Check sheet for the modelled part. Datum: model origin and axes. Units: mm. A direction names the side the tool comes from. Give positions to 0.01 mm unless a question says otherwise; leave off trailing zeros. Loops run counter-clockwise (first coordinate to the right, second up) from the corner with the lowest first, then second, coordinate; pieces in that order, holes last. Notation, with made-up numbers: (9, 5.25) -> (54, 5.25) arc R24 cw to (54, 38.25) -> close; hole circle Ø5 at (15.25, 4). An arc over 180 degrees is marked (long way). Write each question's results on one line, items separated by ' | '. Start each with the question number.
Item 1: Mould release check, pull along X, two halves, no side actions. Record for faces 1 (the face through (73.11, 0.164, -48.295)), 2 (the face through (0.724, 0.515, -49.236)), 3 (the face through (40, 0, -25)): pulls with the +X half, pulls with the -X half, needs draft (parallel to the pull), parting line crosses it, or undercut.
Item 2: Cross-section at A-A on x = 16.4. Enter the section's corners in (y, z).
Item 3: Cross-section at B-B on y = 0.5. State how many separate pieces and enclosed holes the cut face has, then the cut area to 3 significant figures.
Item 4: Gauge pin test, flat ends, axial feed: pin 1 Ø2.5 at (x, z) = (73, -4.5) entering from -Y; pin 2 Ø22 at (x, z) = (14.5, -38.5) entering from -Y. Record the tip position at first contact, or that the pin passes through.
Item 5: Access from +Z, -Z, +X, -X, +Y, -Y to the whole of each face (thin tool, end or side, straight path). Record for faces 4 (the face through (4, 0.333, -4)), 5 (the face through (77.236, 0.515, -0.724)).
Item 6: Scan lines: line 1 along Z through (x, y) = (16.4, 0.45); line 2 along Z through (x, y) = (49.5, 0.25); line 3 along Z through (x, y) = (7.5, 0.3). Record each from-to range of solid material in increasing order.
Item 7: Cross-section at C-C on z = -19. Enter the section's corners in (x, y), then the cut area to 3 significant figures.
from build123d import *

# Parameters (mm, degrees)
SKETCH1_W                   = 78
SKETCH1_H                   = 50
STEEL_FACE_DEPTH            = 1.016
CARD_EDGES_R                = 2.54
SKETCH2_R                   = 2.54
MAGNET_CAVITY_DEPTH         = 0.333375
MIRROR2_COPY_1_SKETCH_R     = 2.54
MIRROR2_COPY_1_DEPTH        = 0.333375
SKETCH3_R                   = 10.049999966
BATTERY_POCKETS_DEPTH       = 0.873000032
SKETCH5_W                   = 35.000000104
SKETCH5_H                   = 3.000000096
LED_SLOT_DEPTH              = 93.655449144
LED_SLOT_CORNER_ROUND_R     = 1.27
LED_SLOT_SURFACE_ROUND_R    = 0.127
SKETCH6_W                   = 2.59999988
SKETCH6_H                   = 3.000000096
ALS_DATA_SENSOR_SLOT_DEPTH  = 93.655449144
SKETCH8_W                   = 2.59999988
SKETCH8_H                   = 3.000000096
ALS_CLOCK_SENSOR_SLOT_DEPTH = 93.655449144
FILLET4_SIZE                = 1.27


with BuildPart() as part:
    # Sketch1 → steel_face (new body)
    with BuildSketch(Plane(origin=(0, 0, 0), x_dir=(1, 0, 0), z_dir=(0, 1, 0))):
        with Locations((39, 25)):
            Rectangle(SKETCH1_W, SKETCH1_H)
    extrude(amount=STEEL_FACE_DEPTH)

    # card_edges
    card_edges_edges = [part.edges().sort_by_distance(p)[0] for p in [
        (0, 0.508, -50),
        (78, 0.508, -50),
        (78, 0.508, 0),
        (0, 0.508, 0),
    ]]
    fillet(card_edges_edges, radius=CARD_EDGES_R)

    # Sketch2 → magnet_cavity (cut)
    with BuildSketch(Plane.XZ):
        with Locations(Location((4.1275, -45.8725, 0), (0, 0, 270))):
            Circle(SKETCH2_R)
    magnet_cavity = extrude(amount=-MAGNET_CAVITY_DEPTH, mode=Mode.SUBTRACT)

    # Mirror1: magnet_cavity across plane
    add(magnet_cavity.mirror(Plane.XY.offset(-25.000000038)), mode=Mode.SUBTRACT)

    # Mirror2: magnet_cavity across plane
    add(magnet_cavity.mirror(Plane(origin=(38.999999978, 0, 0), x_dir=(0, 0, 1), z_dir=(1, 0, 0))), mode=Mode.SUBTRACT)

    # Mirror2 copy 1 sketch → Mirror2 copy 1 (cut)
    with BuildSketch(Plane(origin=(77.999999956, 0, -50.000000076), x_dir=(-1, 0, 0), z_dir=(0, -1, 0))):
        with Locations(Location((4.1275, -45.8725, 0), (0, 0, 270))):
            Circle(MIRROR2_COPY_1_SKETCH_R)
    extrude(amount=-MIRROR2_COPY_1_DEPTH, mode=Mode.SUBTRACT)

    # Sketch3 → battery_pockets (cut)
    with BuildSketch(Plane.XZ):
        with Locations(Location((16.399999966, -11.637499966, 0), (0, 0, 270))):
            Circle(SKETCH3_R)
        with Locations(Location((16.399999966, -38.362500034, 0), (0, 0, 270))):
            Circle(SKETCH3_R)
    extrude(amount=-BATTERY_POCKETS_DEPTH, mode=Mode.SUBTRACT)

    # Sketch5 → led_slot (cut, through all)
    with BuildSketch(Plane(origin=(0, 0, 0), x_dir=(1, 0, 0), z_dir=(0, 1, 0))):
        with Locations((58.912499948, 25.000000038)):
            Rectangle(SKETCH5_W, SKETCH5_H)
    extrude(amount=LED_SLOT_DEPTH, mode=Mode.SUBTRACT)

    # led_slot_corner_round
    led_slot_corner_round_edges = [part.edges().sort_by_distance(p)[0] for p in [
        (76.4125, 0.508, -23.49999999),
        (76.4125, 0.508, -26.500000086),
        (41.412499896, 0.508, -26.500000086),
        (41.412499896, 0.508, -23.49999999),
    ]]
    fillet(led_slot_corner_round_edges, radius=LED_SLOT_CORNER_ROUND_R)

    # led_slot_surface_round
    led_slot_surface_round_edges = [part.edges().sort_by_distance(p)[0] for p in [
        (58.912499948, 1.016, -26.500000086),
        (41.412499896, 1.016, -25.000000038),
        (58.912499948, 1.016, -23.49999999),
        (76.4125, 1.016, -25.000000038),
        (41.784474284, 1.016, -26.128025698),
        (41.784474284, 1.016, -23.871974378),
        (76.040525612, 1.016, -26.128025698),
        (76.040525612, 1.016, -23.871974378),
    ]]
    fillet(led_slot_surface_round_edges, radius=LED_SLOT_SURFACE_ROUND_R)

    # Sketch6 → als_data_sensor_slot (cut, through all)
    with BuildSketch(Plane.XZ):
        with Locations((2.88749994, -25.000000038)):
            Rectangle(SKETCH6_W, SKETCH6_H)
    extrude(amount=-ALS_DATA_SENSOR_SLOT_DEPTH, mode=Mode.SUBTRACT)

    # Sketch8 → als_clock_sensor_slot (cut, through all)
    with BuildSketch(Plane.XZ):
        with Locations((36.112500038, -25.000000038)):
            Rectangle(SKETCH8_W, SKETCH8_H)
    extrude(amount=-ALS_CLOCK_SENSOR_SLOT_DEPTH, mode=Mode.SUBTRACT)

    # Fillet4
    # a fillet whose section is not a circle: 1.27 mm, written as the material it adds along each edge
    with BuildSketch(Plane(origin=(1.5875, 0, -26.500000086), x_dir=(0, 0, 1), z_dir=(0, 1, 0)), Plane(origin=(1.5875, 0, -23.49999999), x_dir=(1, 0, 0), z_dir=(0, 1, 0)), Plane(origin=(34.812500098, 0, -23.49999999), x_dir=(1, 0, 0), z_dir=(0, 1, 0))) as fillet4_piece_1:
        with BuildLine():
            add(Edge.make_bspline([(FILLET4_SIZE, 0), (FILLET4_SIZE * 0.831801948466, 0), (FILLET4_SIZE * 0.663603896932, 0), (FILLET4_SIZE * 0.292893218813, FILLET4_SIZE * 0.0716919198361), (FILLET4_SIZE * 0.0716919198361, FILLET4_SIZE * 0.292893218813), (0, FILLET4_SIZE * 0.663603896932), (0, FILLET4_SIZE * 0.831801948466), (0, FILLET4_SIZE)], knots=[0, 0, 0, 0, 0, 0, 0.5, 0.5, 1, 1, 1, 1, 1, 1], degree=5))
            Line((0, FILLET4_SIZE), (-FILLET4_SIZE * 0.02, FILLET4_SIZE))
            Line((-FILLET4_SIZE * 0.02, FILLET4_SIZE), (-FILLET4_SIZE * 0.02, -FILLET4_SIZE * 0.02))
            Line((-FILLET4_SIZE * 0.02, -FILLET4_SIZE * 0.02), (FILLET4_SIZE, -FILLET4_SIZE * 0.02))
            Line((FILLET4_SIZE, -FILLET4_SIZE * 0.02), (FILLET4_SIZE, 0))
        make_face()
    extrude(amount=1.016)
    with BuildSketch(Plane(origin=(4.18749988, 0, -26.500000086), x_dir=(0, 0, 1), z_dir=(0, 1, 0)), Plane(origin=(4.18749988, 0, -23.49999999), x_dir=(-1, 0, 0), z_dir=(0, 1, 0)), Plane(origin=(34.812500098, 0, -26.500000086), x_dir=(1, 0, 0), z_dir=(0, 1, 0)), Plane(origin=(37.412499978, 0, -26.500000086), x_dir=(0, 0, 1), z_dir=(0, 1, 0)), Plane(origin=(37.412499978, 0, -23.49999999), x_dir=(-1, 0, 0), z_dir=(0, 1, 0))) as fillet4_piece_2:
        with BuildLine():
            add(Edge.make_bspline([(FILLET4_SIZE, 0), (FILLET4_SIZE * 0.831801948466, 0), (FILLET4_SIZE * 0.663603896932, 0), (FILLET4_SIZE * 0.292893218813, -FILLET4_SIZE * 0.0716919198361), (FILLET4_SIZE * 0.0716919198361, -FILLET4_SIZE * 0.292893218813), (0, -FILLET4_SIZE * 0.663603896932), (0, -FILLET4_SIZE * 0.831801948466), (0, -FILLET4_SIZE)], knots=[0, 0, 0, 0, 0, 0, 0.5, 0.5, 1, 1, 1, 1, 1, 1], degree=5))
            Line((0, -FILLET4_SIZE), (-FILLET4_SIZE * 0.02, -FILLET4_SIZE))
            Line((-FILLET4_SIZE * 0.02, -FILLET4_SIZE), (-FILLET4_SIZE * 0.02, FILLET4_SIZE * 0.02))
            Line((-FILLET4_SIZE * 0.02, FILLET4_SIZE * 0.02), (FILLET4_SIZE, FILLET4_SIZE * 0.02))
            Line((FILLET4_SIZE, FILLET4_SIZE * 0.02), (FILLET4_SIZE, 0))
        make_face()
    extrude(amount=1.016)


solid = part.part
Answer sheet:
1) face 1: undercut | face 2: pulls with the -X half | face 3: needs draft
2) outline: (0, -50) -> (1.02, -50) -> (1.02, 0) -> (0, 0) -> (0, -1.59) -> (0.87, -1.59) -> (0.87, -21.69) -> (0, -21.69) -> (0, -28.31) -> (0.87, -28.31) -> (0.87, -48.41) -> (0, -48.41) -> close
3) separate pieces: 1 | enclosed holes: 5 | area: 3,140 mm²
4) pin 1: stops at y = 0.33 | pin 2: stops at y = 0
5) face 4: -Y | face 5: +Z, +X, +Y, -Y
6) line 1: z = -50 to -48.41, -28.31 to -21.69, -1.59 to 0 | line 2: z = -50 to -26.5, -23.5 to 0 | line 3: z = -50 to -43.03, -33.69 to -16.31, -6.97 to 0
7) outline: (0, 0) -> (9.56, 0) -> (9.56, 0.87) -> (23.24, 0.87) -> (23.24, 0) -> (78, 0) -> (78, 1.02) -> (0, 1.02) -> close | area: 67.3 mm²
